from build123d import *

# Parameters (mm, degrees)
SKETCH2_W          = 2.386092155
SKETCH2_H          = 2.248872797
CUT_EXTRUDE1_DEPTH = 3
SKETCH3_W          = 2.355598965
SKETCH3_H          = 2.325105774
CUT_EXTRUDE2_DEPTH = 4


with BuildPart() as part:
    # Sketch1 → Revolve1 (revolve)
    with BuildSketch(Plane.XY, mode=Mode.PRIVATE) as revolve1_sk:
        Polygon((-116.835752997, 27.175404574), (-105.835752997, 27.175404574), (-105.835752997, 28.175404574), (-103.835752997, 28.175404574), (-103.835752997, 26.175404574), (-116.835752997, 26.175404574), align=None)
    revolve(revolve1_sk.sketch.rotate(Axis((-116.835752997, 26.175404574, 0), (1, 0, 0)), 90), axis=Axis((-116.835752997, 26.175404574, 0), (1, 0, 0)))

    # Sketch2 → Cut-Extrude1 (cut)
    with BuildSketch(Plane.ZY.offset(116.835752997)):
        with Locations((0.019058245, 26.198274467)):
            Rectangle(SKETCH2_W, SKETCH2_H)
    extrude(amount=-CUT_EXTRUDE1_DEPTH, mode=Mode.SUBTRACT)

    # Sketch3 → Cut-Extrude2 (cut)
    with BuildSketch(Plane.ZY.offset(113.835752997)):
        with Locations((-0.034304839, 26.259260848)):
            Rectangle(SKETCH3_W, SKETCH3_H)
    extrude(amount=-CUT_EXTRUDE2_DEPTH, mode=Mode.SUBTRACT)


solid = part.part
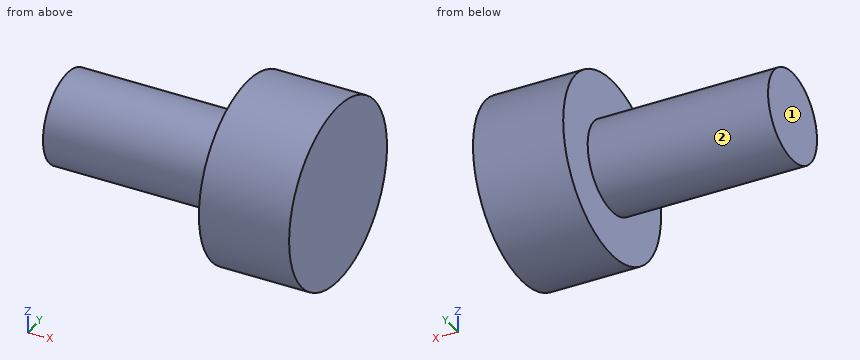
The model under review builds one solid part; all positions refer to its coordinate system, in mm. Face numbers are marked on the shaded views. A direction names the side the tool comes from. Give positions to 0.01 mm unless a question says otherwise; leave off trailing zeros. Loops run counter-clockwise (first coordinate to the right, second up) from the corner with the lowest first, then second, coordinate; pieces in that order, holes last. Notation, with made-up numbers: (39, 24.25) -> (67, 24.25) arc R27 ccw to (67, 59.25) -> close; hole circle Ø2 at (87.25, 40.25). An arc over 180 degrees is marked (long way). Answer as a JSON object with one key per item and string values. Group by question number.
Q1. Wall thickness on line 1 along X through (y, z) = (25.05, -0.15); line 2 along Y through (x, z) = (-105.45, 0.1); line 3 along Y through (x, z) = (-104.2, 1.25): over which ranges is each line inside the solid? List them lowest first.
Q2. Take a section at C-C (x = -104.3). Write out the cut boundary in (y, z), plus the area to 3 significant figures.
Q3. Take a section at B-B (y = 26.25). Write out the cut boundary in (x, z), plus the area to 3 significant figures.
Q4. Tool access review of the marked faces 1 and 2: name each direction out of +Z, -Z, +X, -X, +Y, -Y from which nothing blocks a thin tool from reaching the whole face with its end or side.
Q5. Insertion check: pin 1 (1.5 mm diameter, centred on x = -107, z = -0.5, fed in from -Y). The pin has a flat end and moves straight along its axis. Give the tip position at first contact, or say it passes through.
Q6. Take a section at D-D (z = 1.15). Write out the cut boundary in (x, y), plus the area to 3 significant figures.
Q7. Take a section at A-A (z = 0). Write out the cut boundary in (x, y), plus the area to 3 significant figures.
Answer below:
{
 "1": {"line 1": "x = -105.84 to -103.84", "line 2": "y = 24.18 to 28.17", "line 3": "y = 24.61 to 27.74"},
 "2": {"outline": "circle Ø4 at (26.18, 0)", "area": "12.6 mm2"},
 "3": {"outline": "(-109.84, -1) -> (-105.84, -1) -> (-105.84, -2) -> (-103.84, -2) -> (-103.84, 2) -> (-105.84, 2) -> (-105.84, 1) -> (-109.84, 1) -> close", "area": "16.0 mm2"},
 "4": {"face 1": "+Z, -Z, -X, +Y, -Y", "face 2": "-X"},
 "5": {"pin 1": "stops at y = 25.18"},
 "6": {"outline": "(-105.84, 24.54) -> (-103.84, 24.54) -> (-103.84, 27.81) -> (-105.84, 27.81) -> close", "area": "6.55 mm2"},
 "7": {"outline": "(-109.84, 25.18) -> (-105.84, 25.18) -> (-105.84, 24.18) -> (-103.84, 24.18) -> (-103.84, 28.18) -> (-105.84, 28.18) -> (-105.84, 27.18) -> (-109.84, 27.18) -> close", "area": "16.0 mm2"}
}
